Check sheet for the modelled part. Datum: model origin and axes. Units: mm. Face numbers are marked on the shaded views. A direction names the side the tool comes from. Coordinates: 2 decimals unless noted, no trailing zeros. Write each loop counter-clockwise with the first axis right and the second up, starting at its lowest first coordinate (ties: lowest second). Pieces come first, ordered by that corner, then holes. Notation, with made-up numbers: M -8,59.5 L 11,59.5 A30 ccw 11,90.5 Z; hole C -29.5,80.5 d1. An arc over 180 degrees is marked long. Answer as CSV lines item,"result".
from build123d import *

# Parameters (mm, degrees)
F0_W     = 31.79
F0_H     = 10
F1_DEPTH = 14.9
F2_W     = 28.787708
F2_H     = 12.56
F3_DEPTH = 8.5
F4_R     = 2
F5_DEPTH = 2
F6_R     = 3.25
F7_DEPTH = 8.5
F8_R     = 2.8
F9_DEPTH = 8.5


with BuildPart() as f1:
    # F0 (on Front) → F1 (new body)
    with BuildSketch(Plane.XZ):
        with Locations((-0.331146, 0)):
            Rectangle(F0_W, F0_H)
    extrude(amount=F1_DEPTH)

    # F2 (on face) → F3 (cut)
    with BuildSketch(Plane(origin=(0, 0, -5), x_dir=(1, 0, 0), z_dir=(0, 0, -1))):
        with Locations((0, 7.45)):
            Rectangle(F2_W, F2_H)
    extrude(amount=-F3_DEPTH, mode=Mode.SUBTRACT)

    # F4 (on face) → F5 (join)
    with BuildSketch(Plane.XY.offset(5)):
        with Locations((-12.381146, -3.845)):
            Circle(F4_R)
        with Locations((-4.331169, -3.825617)):
            Circle(F4_R)
        with Locations((3.718807, -3.806234)):
            Circle(F4_R)
        with Locations((11.718854, -3.824759)):
            Circle(F4_R)
        with Locations((-12.381146, -11.055)):
            Circle(F4_R)
        with Locations((-4.331169, -10.990121)):
            Circle(F4_R)
        with Locations((3.718807, -10.925242)):
            Circle(F4_R)
        with Locations((11.718854, -10.890886)):
            Circle(F4_R)
    extrude(amount=F5_DEPTH)

    # F6 (on face) → F7 (join)
    with BuildSketch(Plane(origin=(0, 0, 3.5), x_dir=(1, 0, 0), z_dir=(0, 0, -1))):
        with Locations((-0.017932, 6.96)):
            Circle(F6_R)
        with Locations((-7.847932, 6.96)):
            Circle(F6_R)
        with Locations((7.812068, 6.96)):
            Circle(F6_R)
    extrude(amount=F7_DEPTH)

    # F8 (on face) → F9 (cut)
    with BuildSketch(Plane(origin=(0, 0, -5), x_dir=(1, 0, 0), z_dir=(0, 0, -1))):
        with Locations((-7.847932, 6.96)):
            Circle(F8_R)
        with Locations((0, 6.96)):
            Circle(F8_R)
        with Locations((7.812068, 6.96)):
            Circle(F8_R)
    extrude(amount=-F9_DEPTH, mode=Mode.SUBTRACT)


solid = f1.part
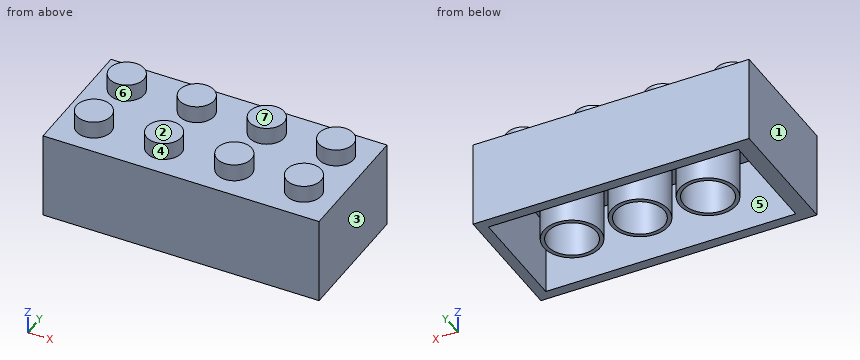
1) Section check C-C, the plane z = 5.5. Record the boundary of the cut face in (x, y) (3 decimals), plus the area to 3 significant figures.
Answer key:
outline,"C -12.381,-11.055 d4; C -12.381,-3.845 d4; C -4.331,-10.99 d4; C -4.331,-3.826 d4; C 3.719,-10.925 d4; C 3.719,-3.806 d4; C 11.719,-10.891 d4; C 11.719,-3.825 d4"
area,"101 mm2"
2) Depth check by flat-ended pin: P1, Ø4.5, axis at x = 7.81, y = -6.96, coming from the +Z side; P2, Ø3, axis at x = 7.5, y = -7, coming from the -Z side. Enter the tip coordinate at first touch or a pass-through.
Answer key:
P1,"stops at z = 5"
P2,"stops at z = 3.5"
3) Section check A-A, the plane z = 1.75. Record the boundary of the cut face in (x, y), plus the area to 3 significant figures.
Answer key:
outline,"M -16.23,-14.9 L 15.56,-14.9 L 15.56,0 L -16.23,0 Z; C -7.85,-6.96 d6.5; C -0.02,-6.96 d6.5; C 7.81,-6.96 d6.5; hole M -14.39,-13.73 L 14.39,-13.73 L 14.39,-1.17 L -14.39,-1.17 Z; hole C -7.85,-6.96 d5.6; hole C 0,-6.96 d5.6; hole C 7.81,-6.96 d5.6"
area,"138 mm2"
4) Tool access check on the marked faces 5, 6 and 7. Record the directions out of +Z, -Z, +X, -X, +Y, -Y that give a thin tool (end or side, any length) a straight path to the whole face; none if there is none.
Answer key:
face 5,"-Z"
face 6,"+Z"
face 7,"+Z, +X, -X, +Y, -Y"
5) Thickness scan on line 1 along Y through (x, z) = (0, 0); line 2 along Y through (x, z) = (-7, 0); line 3 along X through (y, z) = (-1.5, 2). Record the ranges inside material, lowest first.
Answer key:
line 1,"y = -14.9 to -13.73, -10.21 to -9.76, -4.16 to -3.71, -1.17 to 0"
line 2,"y = -14.9 to -13.73, -10.1 to -9.63, -4.29 to -3.82, -1.17 to 0"
line 3,"x = -16.23 to -14.39, 14.39 to 15.56"
6) Mould release check, pull along X, two halves, no side actions. Record for the marked faces 1, 2, 3 and 4: pulls with the +X half, pulls with the -X half, needs draft (parallel to the pull), parting line crosses it, or undercut.
Answer key:
face 1,"pulls with the -X half"
face 2,"needs draft"
face 3,"pulls with the +X half"
face 4,"undercut"
7) Section check D-D, the plane x = 0. Record the boundary of the cut face in (y, z).
Answer key:
outline,"M -14.9,-5 L -13.73,-5 L -13.73,3.5 L -10.21,3.5 L -10.21,-5 L -9.76,-5 L -9.76,3.5 L -4.16,3.5 L -4.16,-5 L -3.71,-5 L -3.71,3.5 L -1.17,3.5 L -1.17,-5 L 0,-5 L 0,5 L -14.9,5 Z"
